from build123d import *

# Parameters (mm, degrees)
F0_R     = 7
F1_DEPTH = 3


with BuildPart() as f1:
    # F0 (on Top) → F1 (new body)
    with BuildSketch(Plane.XY):
        with BuildLine():
            ThreePointArc((30, 16), (25.8994949366, 25.8994949366), (16, 30))
            Line((16, 30), (-16, 30))
            ThreePointArc((-16, 30), (-25.8994949366, 25.8994949366), (-30, 16))
            Line((-30, 16), (-30, -16))
            ThreePointArc((-30, -16), (-25.8994949366, -25.8994949366), (-16, -30))
            Line((-16, -30), (16, -30))
            ThreePointArc((16, -30), (25.8994949366, -25.8994949366), (30, -16))
            Line((30, -16), (30, 16))
        make_face()
        with BuildLine():
            Line((19.8875351453, -5.2301914546), (18.2880349891, 5.685147502))
            Line((18.2880349891, 5.685147502), (21.1683848797, 5.685147502))
            Line((21.1683848797, 5.685147502), (21.7150890347, 0.6273530628))
            add(Edge.make_bspline(
                [(21.7150890347, 0.6273530628), (21.8494220556, -0.5628999831), (21.8494220556, -2.2342526854)],
                knots=[0, 0, 0, 1, 1, 1], degree=2))
            Line((21.8494220556, -2.2342526854), (21.9087785067, -2.2342526854))
            add(Edge.make_bspline(
                [(21.9087785067, -2.2342526854), (22.1055920025, -1.7344088866), (22.3398937832, -1.0658678057)],
                knots=[0, 0, 0, 1, 1, 1], degree=2))
            add(Edge.make_bspline(
                [(22.3398937832, -1.0658678057), (22.5741955639, -0.3973267248), (22.9740706029, 0.4336635907)],
                knots=[0, 0, 0, 1, 1, 1], degree=2))
            Line((22.9740706029, 0.4336635907), (25.5107778819, 5.685147502))
            Line((25.5107778819, 5.685147502), (28.7035301468, 5.685147502))
            Line((28.7035301468, 5.685147502), (22.0649796938, -6.7922033259))
            add(Edge.make_bspline(
                [(22.0649796938, -6.7922033259), (20.3373945642, -10.0349399707), (17.3508278663, -10.0349399707)],
                knots=[0, 0, 0, 1, 1, 1], degree=2))
            add(Edge.make_bspline(
                [(17.3508278663, -10.0349399707), (16.4698531709, -10.0349399707), (15.9137769447, -9.8474985461)],
                knots=[0, 0, 0, 1, 1, 1], degree=2))
            Line((15.9137769447, -9.8474985461), (15.9137769447, -7.5044807392))
            add(Edge.make_bspline(
                [(15.9137769447, -7.5044807392), (16.5791940019, -7.6325657126), (17.0477975633, -7.6325657126)],
                knots=[0, 0, 0, 1, 1, 1], degree=2))
            add(Edge.make_bspline(
                [(17.0477975633, -7.6325657126), (17.8662917838, -7.6325657126), (18.4864104967, -7.1639621512)],
                knots=[0, 0, 0, 1, 1, 1], degree=2))
            add(Edge.make_bspline(
                [(18.4864104967, -7.1639621512), (19.1065292096, -6.6953585898), (19.6344892221, -5.7081670872)],
                knots=[0, 0, 0, 1, 1, 1], degree=2))
            Line((19.6344892221, -5.7081670872), (19.8875351453, -5.2301914546))
        make_face(mode=Mode.SUBTRACT)
        with BuildLine():
            Line((-26.4667291471, 9.0434730253), (-22.305529522, 9.0434730253))
            add(Edge.make_bspline(
                [(-22.305529522, 9.0434730253), (-20.0718525461, 9.0434730253), (-18.9300218682, 8.2468469709)],
                knots=[0, 0, 0, 1, 1, 1], degree=2))
            add(Edge.make_bspline(
                [(-18.9300218682, 8.2468469709), (-17.7881911903, 7.4502209166), (-17.7881911903, 5.8694649028)],
                knots=[0, 0, 0, 1, 1, 1], degree=2))
            add(Edge.make_bspline(
                [(-17.7881911903, 5.8694649028), (-17.7881911903, 4.4042977676), (-18.5973133396, 3.4530325379)],
                knots=[0, 0, 0, 1, 1, 1], degree=2))
            add(Edge.make_bspline(
                [(-18.5973133396, 3.4530325379), (-19.4064354889, 2.5017673083), (-20.8997188379, 2.1893649341)],
                knots=[0, 0, 0, 1, 1, 1], degree=2))
            Line((-20.8997188379, 2.1893649341), (-20.8997188379, 2.130008483))
            add(Edge.make_bspline(
                [(-20.8997188379, 2.130008483), (-19.9250234302, 1.8769625598), (-19.3439550141, 1.1881153246)],
                knots=[0, 0, 0, 1, 1, 1], degree=2))
            add(Edge.make_bspline(
                [(-19.3439550141, 1.1881153246), (-18.7628865979, 0.4992680893), (-18.7628865979, -0.5722720544)],
                knots=[0, 0, 0, 1, 1, 1], degree=2))
            add(Edge.make_bspline(
                [(-18.7628865979, -0.5722720544), (-18.7628865979, -2.8090730541), (-20.2561699469, -4.0196322543)],
                knots=[0, 0, 0, 1, 1, 1], degree=2))
            add(Edge.make_bspline(
                [(-20.2561699469, -4.0196322543), (-21.7494532958, -5.2301914546), (-24.3861293346, -5.2301914546)],
                knots=[0, 0, 0, 1, 1, 1], degree=2))
            Line((-24.3861293346, -5.2301914546), (-29.4814120587, -5.2301914546))
            Line((-29.4814120587, -5.2301914546), (-26.4667291471, 9.0434730253))
        make_face(mode=Mode.SUBTRACT)
        with BuildLine():
            add(Edge.make_bspline(
                [(-10.521711965, -3.8150086992), (-11.8306779132, -5.4270049503), (-13.6363636364, -5.4270049503)],
                knots=[0, 0, 0, 1, 1, 1], degree=2))
            add(Edge.make_bspline(
                [(-13.6363636364, -5.4270049503), (-15.073414558, -5.4270049503), (-15.898156826, -4.3867050441)],
                knots=[0, 0, 0, 1, 1, 1], degree=2))
            add(Edge.make_bspline(
                [(-15.898156826, -4.3867050441), (-16.722899094, -3.3464051378), (-16.722899094, -1.4719908922)],
                knots=[0, 0, 0, 1, 1, 1], degree=2))
            add(Edge.make_bspline(
                [(-16.722899094, -1.4719908922), (-16.722899094, 0.4617798044), (-16.019993752, 2.214357124)],
                knots=[0, 0, 0, 1, 1, 1], degree=2))
            add(Edge.make_bspline(
                [(-16.019993752, 2.214357124), (-15.3170884099, 3.9669344436), (-14.1736957201, 4.9275717444)],
                knots=[0, 0, 0, 1, 1, 1], degree=2))
            add(Edge.make_bspline(
                [(-14.1736957201, 4.9275717444), (-13.0303030303, 5.8882090453), (-11.6651046548, 5.8882090453)],
                knots=[0, 0, 0, 1, 1, 1], degree=2))
            add(Edge.make_bspline(
                [(-11.6651046548, 5.8882090453), (-10.7185254608, 5.8882090453), (-10.0296782256, 5.478961935)],
                knots=[0, 0, 0, 1, 1, 1], degree=2))
            add(Edge.make_bspline(
                [(-10.0296782256, 5.478961935), (-9.3408309903, 5.0697148247), (-8.9597000937, 4.2887088891)],
                knots=[0, 0, 0, 1, 1, 1], degree=2))
            Line((-8.9597000937, 4.2887088891), (-8.8815995002, 4.2887088891))
            Line((-8.8815995002, 4.2887088891), (-8.325523274, 5.685147502))
            Line((-8.325523274, 5.685147502), (-6.0606060606, 5.685147502))
            Line((-6.0606060606, 5.685147502), (-8.3848797251, -5.2301914546))
            Line((-8.3848797251, -5.2301914546), (-10.6216807248, -5.2301914546))
            Line((-10.6216807248, -5.2301914546), (-10.4842236801, -3.8150086992))
            Line((-10.4842236801, -3.8150086992), (-10.521711965, -3.8150086992))
        make_face(mode=Mode.SUBTRACT)
        Polygon((-0.1062168072, 5.685147502), (-2.4211184005, -5.2301914546), (-5.3577007185, -5.2301914546), (-3.045923149, 5.685147502), align=None, mode=Mode.SUBTRACT)
        with BuildLine():
            add(Edge.make_bspline(
                [(-1.1027803811, 7.0409738063), (-2.5773195876, 7.0409738063), (-2.5773195876, 8.2437229472)],
                knots=[0, 0, 0, 1, 1, 1], degree=2))
            add(Edge.make_bspline(
                [(-2.5773195876, 8.2437229472), (-2.5773195876, 9.0903333814), (-2.1134020619, 9.5261346935)],
                knots=[0, 0, 0, 1, 1, 1], degree=2))
            add(Edge.make_bspline(
                [(-2.1134020619, 9.5261346935), (-1.6494845361, 9.9619360056), (-0.7997500781, 9.9619360056)],
                knots=[0, 0, 0, 1, 1, 1], degree=2))
            add(Edge.make_bspline(
                [(-0.7997500781, 9.9619360056), (-0.0874726648, 9.9619360056), (0.2842861606, 9.6589057026)],
                knots=[0, 0, 0, 1, 1, 1], degree=2))
            add(Edge.make_bspline(
                [(0.2842861606, 9.6589057026), (0.6560449859, 9.3558753995), (0.6560449859, 8.7904271021)],
                knots=[0, 0, 0, 1, 1, 1], degree=2))
            add(Edge.make_bspline(
                [(0.6560449859, 8.7904271021), (0.6560449859, 8.0094211665), (0.2264917213, 7.5251974864)],
                knots=[0, 0, 0, 1, 1, 1], degree=2))
            add(Edge.make_bspline(
                [(0.2264917213, 7.5251974864), (-0.2030615433, 7.0409738063), (-1.1027803811, 7.0409738063)],
                knots=[0, 0, 0, 1, 1, 1], degree=2))
        make_face(mode=Mode.SUBTRACT)
        Polygon((6.7385192127, 9.9619360056), (3.5145267104, -5.2301914546), (0.5779443924, -5.2301914546), (3.798812871, 9.9619360056), align=None, mode=Mode.SUBTRACT)
        with BuildLine():
            add(Edge.make_bspline(
                [(15.1515151515, -4.5866425636), (13.4739144017, -5.4270049503), (11.3464542331, -5.4270049503)],
                knots=[0, 0, 0, 1, 1, 1], degree=2))
            add(Edge.make_bspline(
                [(11.3464542331, -5.4270049503), (9.2939706342, -5.4270049503), (8.1615120275, -4.3226625573)],
                knots=[0, 0, 0, 1, 1, 1], degree=2))
            add(Edge.make_bspline(
                [(8.1615120275, -4.3226625573), (7.0290534208, -3.2183201643), (7.0290534208, -1.2064488741)],
                knots=[0, 0, 0, 1, 1, 1], degree=2))
            add(Edge.make_bspline(
                [(7.0290534208, -1.2064488741), (7.0290534208, 0.8116704636), (7.8350515464, 2.4767751184)],
                knots=[0, 0, 0, 1, 1, 1], degree=2))
            add(Edge.make_bspline(
                [(7.8350515464, 2.4767751184), (8.641049672, 4.1418797732), (10.0171821306, 5.0150444092)],
                knots=[0, 0, 0, 1, 1, 1], degree=2))
            add(Edge.make_bspline(
                [(10.0171821306, 5.0150444092), (11.3933145892, 5.8882090453), (13.1302717901, 5.8882090453)],
                knots=[0, 0, 0, 1, 1, 1], degree=2))
            add(Edge.make_bspline(
                [(13.1302717901, 5.8882090453), (14.8609809435, 5.8882090453), (15.8263042799, 5.0931450028)],
                knots=[0, 0, 0, 1, 1, 1], degree=2))
            add(Edge.make_bspline(
                [(15.8263042799, 5.0931450028), (16.7916276164, 4.2980809603), (16.7916276164, 2.9110144186)],
                knots=[0, 0, 0, 1, 1, 1], degree=2))
            add(Edge.make_bspline(
                [(16.7916276164, 2.9110144186), (16.7916276164, 1.0865845529), (15.1624492346, 0.0962690265)],
                knots=[0, 0, 0, 1, 1, 1], degree=2))
            add(Edge.make_bspline(
                [(15.1624492346, 0.0962690265), (13.5332708529, -0.8940464999), (10.5060918463, -0.8940464999)],
                knots=[0, 0, 0, 1, 1, 1], degree=2))
            Line((10.5060918463, -0.8940464999), (10.0062480475, -0.8940464999))
            Line((10.0062480475, -0.8940464999), (9.987503905, -1.1002320669))
            Line((9.987503905, -1.1002320669), (9.987503905, -1.2970455627))
            add(Edge.make_bspline(
                [(9.987503905, -1.2970455627), (9.987503905, -2.1842683055), (10.4904717276, -2.6966081993)],
                knots=[0, 0, 0, 1, 1, 1], degree=2))
            add(Edge.make_bspline(
                [(10.4904717276, -2.6966081993), (10.9934395501, -3.2089480931), (11.9306466729, -3.2089480931)],
                knots=[0, 0, 0, 1, 1, 1], degree=2))
            add(Edge.make_bspline(
                [(11.9306466729, -3.2089480931), (12.7803811309, -3.2089480931), (13.4739144017, -3.0230686804)],
                knots=[0, 0, 0, 1, 1, 1], degree=2))
            add(Edge.make_bspline(
                [(13.4739144017, -3.0230686804), (14.1674476726, -2.8371892677), (15.1515151515, -2.3685857064)],
                knots=[0, 0, 0, 1, 1, 1], degree=2))
            Line((15.1515151515, -2.3685857064), (15.1515151515, -4.5866425636))
        make_face(mode=Mode.SUBTRACT)
        with Locations((0, 19.8741126806)):
            Circle(F0_R, mode=Mode.SUBTRACT)
    extrude(amount=F1_DEPTH)


solid = f1.part
The model under review builds one solid part; all positions refer to its coordinate system, in mm. A direction names the side the tool comes from. Give positions to 0.01 mm unless a question says otherwise; leave off trailing zeros. Answer as a JSON object with one key per item and string values. Group by question number.
Q1. Insertion check: pin 1 (8 mm diameter, centred on x = 11.5, y = 5, fed in from +Z); pin 2 (0.9 mm diameter, centred on x = -23.5, z = 1.5, fed in from -Y); pin 3 (0.9 mm diameter, centred on x = -26, z = 2, fed in from +Y); pin 4 (1.5 mm diameter, centred on y = -17, z = 1, fed in from -X). Each pin has a flat end and moves straight along its axis. Give the tip position at first contact, or say it passes through.
Q2. Tool access review of faces 4 (the cylindrical face through (26, 25.8, 1.5)), 5 (the flat face through (-4.22, 0.15, 1.48)): name each direction out of +Z, -Z, +X, -X, +Y, -Y from which nothing blocks a thin tool from reaching the whole face with its end or side.
Q3. Draft analysis for pull direction Y (two halves, no side actions). For faces 1 (the flat face through (-30, 0, 1)), 2 (the cylindrical face through (25.8, -26, 1.5)), 3 (the flat face through (27, 5.685, 1)), state which applies: pulls with the +Y half, pulls with the -Y half, needs draft (parallel to the pull), parting line crosses it, or undercut.
Q4. Take a section at A-A (z = 1.8). State how many separate pieces and enclosed holes the cut face has, plus the area to 3 significant figures.
Q5. Wall thickness on line 1 along Y through (x, z) = (0, 2.4); line 2 along X through (y, z) = (8, 1.55); line 3 along Y through (x, z) = (27, 0.7): over which ranges is each line inside the solid? List them lowest first.
Answer below:
{
 "1": {"pin 1": "stops at z = 3", "pin 2": "stops at y = -28.1", "pin 3": "stops at y = 26.24", "pin 4": "stops at x = -30"},
 "2": {"face 4": "+Z, -Z, +X, +Y", "face 5": "+Z, -Z"},
 "3": {"face 1": "needs draft", "face 2": "pulls with the -Y half", "face 3": "undercut"},
 "4": {"separate pieces": "1", "enclosed holes": "8", "area": "2,820 mm2"},
 "5": {"line 1": "y = -30 to 7.33, 9.83 to 12.87, 26.87 to 30", "line 2": "x = -30 to -26.69, -18.62 to -2.56, 0.52 to 3.38, 6.32 to 30", "line 3": "y = -24.66 to 2.48, 5.69 to 24.66"}
}
